Input: part model. Units: mm. Frame: model coordinates. Coordinates: 2 decimals unless noted, no trailing zeros. Order: outer loops, then holes, each group sorted by start corner. A loop starts at its lowest first (then second) coordinate and runs counter-clockwise, first axis right, second up. Notation, with made-up numbers: (89.5, 49) - (97.5, 49) arc R16 cw to (97.5, 73) - close; hole circle Ø11 at (-40, 35). An arc over 180 degrees is marked (long way). One line per question, with ' | ' between items.
from build123d import *

# Parameters (mm, degrees)
BOSS_EXTRUDE1_DEPTH = 1.5875
SKETCH2_R           = 6.35
SKETCH2_R_2         = 4.7625
CUT_EXTRUDE1_DEPTH  = 200.339494535


with BuildPart() as part:
    # Sketch1 → Boss-Extrude1 (new body)
    with BuildSketch(Plane.XY):
        with BuildLine():
            Line((-29.004064566, -156.10056159), (-29.004064566, -44.966517074))
            Line((-29.004064566, -44.966517074), (-123.96099627, -44.966517074))
            Line((-123.96099627, -44.966517074), (-119.793452617, -84.639660454))
            ThreePointArc((-119.793452617, -84.639660454), (-99.185042421, -129.235543476), (-55.642806391, -151.98577501))
            Line((-55.642806391, -151.98577501), (-29.004064566, -156.10056159))
        make_face()
    extrude(amount=BOSS_EXTRUDE1_DEPTH)

    # Sketch2 → Cut-Extrude1 (cut, through all)
    with BuildSketch(Plane(origin=(0, 0, 0), x_dir=(-1, 0, 0), z_dir=(0, 0, -1))):
        with Locations((71.892516398, -102.315332665)):
            Circle(SKETCH2_R)
        with Locations((96.475228053, -102.315332665)):
            Circle(SKETCH2_R)
        with Locations((96.475228053, -74.107206632)):
            Circle(SKETCH2_R)
        with Locations((71.892516398, -74.107206632)):
            Circle(SKETCH2_R)
        with Locations((46.831572971, -102.315332665)):
            Circle(SKETCH2_R_2)
        with Locations((46.831572971, -74.107206632)):
            Circle(SKETCH2_R_2)
    extrude(amount=-CUT_EXTRUDE1_DEPTH, mode=Mode.SUBTRACT)


solid = part.part
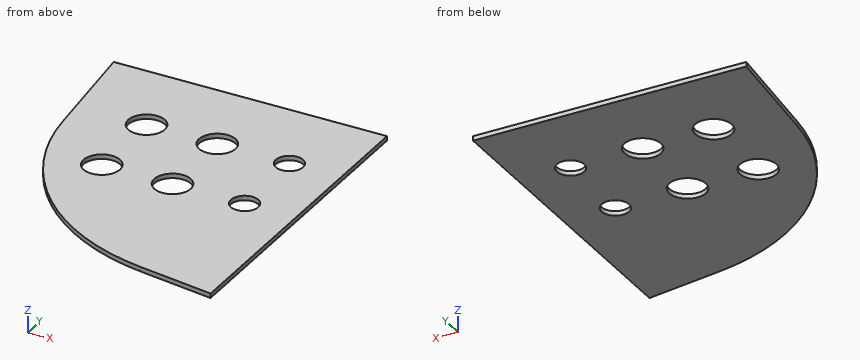
Item 1: Contact query for a flat-ended pin moving along its axis: P1, Ø7.5, axis at x = -96.48, y = -102.32, coming from the +Z side. Output: stop coordinate, or through.
Data:
P1: through
Item 2: Section C-C on x = -97.5. Return the cut outline in (y, z).
Data:
outline: (-130.95, 0) - (-108.58, 0) - (-108.58, 1.59) - (-130.95, 1.59) - close; (-96.05, 0) - (-80.37, 0) - (-80.37, 1.59) - (-96.05, 1.59) - close; (-67.84, 0) - (-44.97, 0) - (-44.97, 1.59) - (-67.84, 1.59) - close
Item 3: Section A-A on x = -76.5. Return the cut outline in (y, z), and give its area (3 significant figures).
Data:
outline: (-145.61, 0) - (-106.68, 0) - (-106.68, 1.59) - (-145.61, 1.59) - close; (-97.95, 0) - (-78.48, 0) - (-78.48, 1.59) - (-97.95, 1.59) - close; (-69.74, 0) - (-44.97, 0) - (-44.97, 1.59) - (-69.74, 1.59) - close | area: 132 mm^2
Item 4: Section D-D on y = -122.5. Return the cut outline in (x, z), and give its area (3 significant figures).
Data:
outline: (-104.89, 0) - (-29, 0) - (-29, 1.59) - (-104.89, 1.59) - close | area: 120 mm^2
Item 5: Ray query, line 1 (X direction, y = -72.5, z = 1.2); line 2 (X direction, y = -107.5, z = 1.55); line 3 (Y direction, x = -70, z = 0.25). Return the intervals inside material, ascending.
Data:
line 1: -121.07 to -102.62, -90.33 to -78.04, -65.75 to -51.31, -42.35 to -29 | line 2: -113.7 to -100.14, -92.81 to -75.56, -68.23 to -29 | line 3: -148.31 to -108.38, -96.25 to -80.17, -68.05 to -44.97
Item 6: Section B-B on z = 0.5. Count the separate pieces of the cut face and the enclosed holes in it, and give its area (3 significant figures).
Data:
separate pieces: 1 | enclosed holes: 6 | area: 8,050 mm^2
